Could you check a few things on this model? Use its own coordinates, in mm. Face numbers are marked on the shaded views. A direction names the side the tool comes from. Coordinates: 2 decimals unless noted, no trailing zeros. Loops run counter-clockwise (first coordinate to the right, second up) from the corner with the lowest first, then second, coordinate; pieces in that order, holes last. Notation, with made-up numbers: (6, 4.25) -> (41, 4.25) arc R24 cw to (41, 17.25) -> close; hole circle Ø10 at (80, 60.5). An arc over 180 degrees is marked (long way). One line per question, with ' | ' between items. Start each with the question number.
(1) Which directions (+Z, -Z, +X, -X, +Y, -Y) give clear straight access to the entire face, cutting with the end or side of a thin tool? Please do the marked faces 4, 5 and 6.
(2) Suppose I cut it at A-A (y = -0.5). Please give me the cut outline in (x, z).
(3) If I drill on line 1 along X through (y, z) = (-4, -5.5); line 2 along Y through (x, z) = (7.5, -10.5); line 3 along Z through (x, y) = (11.5, -1.25), over which ranges is the centre line in solid material (lowest first)?
(4) I'm going to push flat-ended pins straight in: pin 1 Ø0.6 at (y, z) = (-0.5, 15) entering from +X; pin 2 Ø2 at (x, y) = (13, 8.5) entering from -Z; pin 3 Ø1.6 at (x, y) = (4, 9) entering from +Z. Where does each tip first touch, or does it pass through?
(5) Suppose I cut it at B-B (x = 4.75). Please give me the cut outline in (y, z).
(6) Suppose I cut it at C-C (z = -1). Please give me the cut outline in (x, y), plus the area to 3 significant figures.
(7) Suppose I cut it at D-D (y = 7.25). Please give me the cut outline in (x, z), plus the area to 3 significant figures.
(8) If we mould it in two halves opening along Z, with no side actions, what happens to the marked faces 1, 2 and 3? For each: pulls with the +Z half, pulls with the -Z half, needs draft (parallel to the pull), parting line crosses it, or undercut.
```python
from build123d import *

# Parameters (mm, degrees)
EXTRUDE_3_DEPTH     = 20
SKETCH_4_W          = 6
SKETCH_4_H          = 1.997420006
CUT_EXTRUDE_1_DEPTH = 20
EXTRUDE_4_DEPTH     = 8
SKETCH_6_R          = 1
EXTRUDE_5_DEPTH     = 20
SKETCH_7_W          = 16
SKETCH_7_H          = 28.677583324
CUT_EXTRUDE_3_DEPTH = 18
SKETCH_8_W          = 4
SKETCH_8_H          = 6.365219316
CUT_EXTRUDE_4_DEPTH = 10
SKETCH_9_W          = 8
SKETCH_9_H          = 4
CUT_EXTRUDE_5_DEPTH = 10


with BuildPart() as part:
    # 草图3 → 凸台-拉伸3 (new body)
    with BuildSketch(Plane(origin=(0, 0, 0), x_dir=(0, 0, -1), z_dir=(1, 0, 0))):
        with BuildLine():
            Line((-14.292893219, 8.292893219), (4, -10))
            Line((4, -10), (15, -10))
            Line((15, -10), (15, 10))
            Line((15, 10), (-15, 10))
            ThreePointArc((-15, 10), (-15.923879533, 8.617316568), (-14.292893219, 8.292893219))
        make_face()
    extrude(amount=EXTRUDE_3_DEPTH)

    # 草图4 → 切除-拉伸1 (cut)
    with BuildSketch(Plane(origin=(0, 10, 0), x_dir=(1, 0, 0), z_dir=(0, 1, 0))):
        with Locations((3, -15.001289997)):
            Rectangle(SKETCH_4_W, SKETCH_4_H)
        with Locations((17, -15.001289997)):
            Rectangle(SKETCH_4_W, SKETCH_4_H)
    extrude(amount=-CUT_EXTRUDE_1_DEPTH, mode=Mode.SUBTRACT)

    # 草图5 → 凸台-拉伸4 (add)
    with BuildSketch(Plane(origin=(14, 0, 0), x_dir=(0, 0, -1), z_dir=(1, 0, 0))):
        with BuildLine():
            Line((-14, 9), (-14, -9))
            ThreePointArc((-14, -9), (-15, -10), (-16, -9))
            Line((-16, -9), (-16, 9))
            ThreePointArc((-16, 9), (-15, 10), (-14, 9))
        make_face()
    extrude(amount=-EXTRUDE_4_DEPTH)

    # 草图6 → 凸台-拉伸5 (add)
    with BuildSketch(Plane(origin=(20, 0, 0), x_dir=(0, 0, -1), z_dir=(1, 0, 0))):
        with Locations((15, -9)):
            Circle(SKETCH_6_R)
    extrude(amount=-EXTRUDE_5_DEPTH)

    # 草图7 → 切除-拉伸3 (cut)
    with BuildSketch(Plane(origin=(0, 10, 0), x_dir=(1, 0, 0), z_dir=(0, 1, 0))):
        with Locations((10, 2.336211668)):
            Rectangle(SKETCH_7_W, SKETCH_7_H)
    extrude(amount=-CUT_EXTRUDE_3_DEPTH, mode=Mode.SUBTRACT)

    # 草图8 → 切除-拉伸4 (cut)
    with BuildSketch(Plane.XY.offset(16)):
        with Locations((10, -8.182609658)):
            Rectangle(SKETCH_8_W, SKETCH_8_H)
    extrude(amount=-CUT_EXTRUDE_4_DEPTH, mode=Mode.SUBTRACT)

    # 草图9 → 切除-拉伸5 (cut)
    with BuildSketch(Plane(origin=(0, -8, 0), x_dir=(1, 0, 0), z_dir=(0, 1, 0))):
        with Locations((10, 14)):
            Rectangle(SKETCH_9_W, SKETCH_9_H)
    extrude(amount=-CUT_EXTRUDE_5_DEPTH, mode=Mode.SUBTRACT)


solid = part.part
```
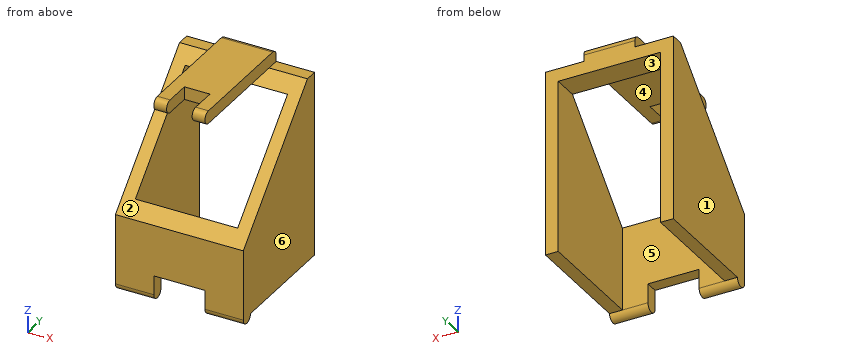
Checks:
1) face 4: +X, -X, -Y | face 5: -Z, +Y | face 6: +Z, -Z, +X, +Y, -Y
2) outline: (0, -15) -> (2, -15) -> (2, 5.5) -> (0, 5.5) -> close; (6, 14) -> (14, 14) -> (14, 16) -> (6, 16) -> close; (18, -15) -> (20, -15) -> (20, 5.5) -> (18, 5.5) -> close
3) line 1: x = 0 to 2, 18 to 20 | line 2: y = -10 to -8 | line 3: z = 14 to 16
4) pin 1: stops at x = 14 | pin 2: stops at z = 12 | pin 3: stops at z = 14
5) outline: (-10, -15) arc R1 ccw to (-8, -15) -> (-8, -2) -> (-10, -4) -> close; (6, 12) -> (10, 12) -> (10, 14) -> (8, 14) -> close
6) outline: (0, -7) -> (2, -7) -> (2, 10) -> (0, 10) -> close; (18, -7) -> (20, -7) -> (20, 10) -> (18, 10) -> close | area: 68.0 mm^2
7) outline: (0, -15) -> (2, -15) -> (2, 12) -> (18, 12) -> (18, -15) -> (20, -15) -> (20, 13.25) -> (0, 13.25) -> close; (6, 14) -> (14, 14) -> (14, 16) -> (6, 16) -> close | area: 149 mm^2
8) face 1: needs draft | face 2: undercut | face 3: pulls with the -Z half
